```python
from build123d import *

# Parameters (mm, degrees)
Y_KSEKLIK_EKSTR_ZYON1_DEPTH = 35
KES_EKSTR_ZYON1_DEPTH       = 35
IZIM3_R                     = 17.5
IZIM3_R_2                   = 15
Y_KSEKLIK_EKSTR_ZYON2_DEPTH = 75
IZIM4_R                     = 7.5
KES_EKSTR_ZYON2_DEPTH       = 28


with BuildPart() as part:
    # Çizim1 → Yükseklik-Ekstrüzyon1 (new body)
    with BuildSketch(Plane.XY):
        with BuildLine():
            Line((-62.217360921, -15), (62.217360921, -15))
            ThreePointArc((62.217360921, -15), (0, -64), (-62.217360921, -15))
        make_face()
    extrude(amount=Y_KSEKLIK_EKSTR_ZYON1_DEPTH)

    # Çizim2 → Kes-Ekstrüzyon1 (cut)
    with BuildSketch(Plane.XY.offset(35)):
        with BuildLine():
            Line((-48.989794856, -25), (48.989794856, -25))
            ThreePointArc((48.989794856, -25), (0, -55), (-48.989794856, -25))
        make_face()
    extrude(amount=-KES_EKSTR_ZYON1_DEPTH, mode=Mode.SUBTRACT)

    # Çizim3 → Yükseklik-Ekstrüzyon2 (add)
    with BuildSketch(Plane(origin=(0, -15, 0), x_dir=(1, 0, 0), z_dir=(0, 1, 0))):
        with Locations(Location((0, -17.5, 0), (0, 0, 270))):
            Circle(IZIM3_R)
        with Locations(Location((0, -17.5, 0), (0, 0, 270))):
            Circle(IZIM3_R_2, mode=Mode.SUBTRACT)
    extrude(amount=Y_KSEKLIK_EKSTR_ZYON2_DEPTH)

    # Çizim4 → Kes-Ekstrüzyon2 (cut)
    with BuildSketch(Plane(origin=(0, -15, 0), x_dir=(1, 0, 0), z_dir=(0, 1, 0))):
        with Locations(Location((0, -17.5, 0), (0, 0, 270))):
            Circle(IZIM4_R)
    extrude(amount=-KES_EKSTR_ZYON2_DEPTH, mode=Mode.SUBTRACT)


solid = part.part
```
Geometry check sheet. Reference: the model listing, model coordinates, mm. A direction names the side the tool comes from. Coordinates: 2 decimals unless noted, no trailing zeros. Loops run counter-clockwise (first coordinate to the right, second up) from the corner with the lowest first, then second, coordinate; pieces in that order, holes last.
Item 1: Go/stop test with flat-tipped pins: pin 1 Ø6 at (x, z) = (-49.5, 25.5) entering from +Y; pin 2 Ø5 at (y, z) = (-47.5, 30) entering from -X; pin 3 Ø13.5 at (x, z) = (0, 17.5) entering from +Y; pin 4 Ø1.5 at (x, y) = (45.5, -14) entering from +Z. Record where each tip stops, or that it passes through.
Item 2: Thickness scan on line 1 (X direction, y = 40, z = 17.5); line 2 (X direction, y = -22.5, z = 17.5); line 3 (Y direction, x = 19, z = 31.5). Record the ranges inside material, lowest first.
Item 3: Sectioned sample at B-B, the plane x = 10.5. Record the boundary of the cut face in (y, z), then the cut area to 3 significant figures.
Item 4: Access from +Z, -Z, +X, -X, +Y, -Y to the whole of each face (thin tool, end or side, straight path). Record for faces 1 (the face through (5, 60, 32)), 2 (the face through (-1, -25, 26)), 3 (the face through (-10.648, 21.975, 3.613)).
Item 5: Sectioned sample at C-C, the plane z = 17.5. Record the boundary of the cut face in (x, y), then the cut area to 3 significant figures.
Item 6: Sectioned sample at A-A, the plane y = -33. Record the boundary of the cut face in (x, z), then the cut area to 3 significant figures.
Item 7: Sectioned sample at D-D, the plane y = -20. Record the boundary of the cut face in (x, z), then the cut area to 3 significant figures.
Item 8: Release check for a two-part mould opening along Z. For faces 4 (the face through (0.66, 21.975, 2.515)), 5 (the face through (1.2, -63.99, 17.26)), 6 (the face through (1, -23, 0)), 7 (the face through (1, -23, 35)) record: released by +Z, released by -Z, zero draft, split by the parting line, or undercut.
Check result:
1. pin 1: stops at y = -15
1. pin 2: stops at x = -45.51
1. pin 3: stops at y = -54.58
1. pin 4: passes through
2. line 1: x = -17.5 to -15, 15 to 17.5
2. line 2: x = -59.91 to -7.5, 7.5 to 59.91
2. line 3: y = -61.11 to -51.61, -25 to -15
3. outline: (-63.13, 0) - (-53.99, 0) - (-53.99, 35) - (-63.13, 35) - close; (-25, 0) - (-15, 0) - (-15, 3.5) - (60, 3.5) - (60, 6.79) - (-15, 6.79) - (-15, 28.21) - (60, 28.21) - (60, 31.5) - (-15, 31.5) - (-15, 35) - (-25, 35) - close
3. area: 1,160 mm2
4. face 1: +Z, -Z, +X, -X, +Y
4. face 2: +Z, -Z
4. face 3: +Y
5. outline: (-62.22, -15) arc R64 ccw to (62.22, -15) - (17.5, -15) - (17.5, 60) - (15, 60) - (15, -15) - (7.5, -15) - (7.5, -25) - (48.99, -25) arc R55 cw to (-48.99, -25) - (-7.5, -25) - (-7.5, -15) - (-15, -15) - (-15, 60) - (-17.5, 60) - (-17.5, -15) - close
5. area: 2,660 mm2
6. outline: (-54.84, 0) - (-44, 0) - (-44, 35) - (-54.84, 35) - close; (44, 0) - (54.84, 0) - (54.84, 35) - (44, 35) - close
6. area: 759 mm2
7. outline: (-60.79, 0) - (60.79, 0) - (60.79, 35) - (-60.79, 35) - close; hole circle Ø15 at (0, 17.5)
7. area: 4,080 mm2
8. face 4: undercut
8. face 5: zero draft
8. face 6: released by -Z
8. face 7: released by +Z
